```python
from build123d import *

# Parameters (mm, degrees)
TALADRO_DE_MARGEN_PARA_M101_D = 11
TALADRO_DE_MARGEN_PARA_M81_D  = 9
MATRIZC1_COUNT                = 4
CROQUIS8_R                    = 17.4
CORTAR_EXTRUIR2_DEPTH         = 70


with BuildPart() as part:
    # Croquis2 → Revolución1 (revolve)
    with BuildSketch(Plane.XY):
        with BuildLine():
            Line((19, 31), (0, 31))
            Line((0, 31), (0, 0))
            Line((0, 0), (110, 0))
            Line((110, 0), (110, 9))
            ThreePointArc((110, 9), (104.142135624, 23.142135624), (90, 29))
            Line((90, 29), (62, 29))
            Line((62, 29), (52, 23))
            Line((52, 23), (47, 3))
            Line((47, 3), (19, 3))
            Line((19, 3), (19, 31))
        make_face()
        with BuildLine():
            Line((110, 0), (0, 0))
            Line((0, 0), (0, -31))
            Line((0, -31), (19, -31))
            Line((19, -31), (19, -3))
            Line((19, -3), (47, -3))
            Line((47, -3), (52, -23))
            Line((52, -23), (62, -29))
            Line((62, -29), (90, -29))
            ThreePointArc((90, -29), (104.142135624, -23.142135624), (110, -9))
            Line((110, -9), (110, 0))
        make_face()
    revolve(axis=Axis((0, 64.768346902, 0), (0, -1, 0)))

    # Taladro de margen para M101 (through all)
    with Locations(Plane(origin=(0, 31, 0), x_dir=(1, 0, 0), z_dir=(0, 1, 0))):
        with Locations((0, 0)):
            Hole(TALADRO_DE_MARGEN_PARA_M101_D / 2)

    # Taladro de margen para M81 (through all)
    with Locations(Plane(origin=(0, 3, 0), x_dir=(1, 0, 0), z_dir=(0, 1, 0))):
        with Locations((0, 34.5)):
            taladro_de_margen_para_m81 = Hole(TALADRO_DE_MARGEN_PARA_M81_D / 2)

    # MatrizC1: Taladro de margen para M81 ×4 about axis
    matrizc1_axis = Axis((0, 0, 0), (0, 1, 0))
    for i in range(1, MATRIZC1_COUNT):
        add(taladro_de_margen_para_m81.rotate(matrizc1_axis, i * 360 / MATRIZC1_COUNT), mode=Mode.SUBTRACT)

    # Croquis8 → Cortar-Extruir2 (cut)
    with BuildSketch(Plane(origin=(0, 31, 0), x_dir=(1, 0, 0), z_dir=(0, 1, 0))):
        Circle(CROQUIS8_R)
    extrude(amount=-CORTAR_EXTRUIR2_DEPTH, mode=Mode.SUBTRACT)


solid = part.part
```
CAD build for the part. Positions are in the model's coordinates, mm. A direction names the side the tool comes from. Round coordinates to 2 decimals unless told otherwise and drop trailing zeros.
Q1. Which spindle directions (+Z, -Z, +X, -X, +Y, -Y) get a long thin tool onto all of the face, cutting with end or side? Do faces 4 (the flat face through (6, 31, -17)), 5 (the cylindrical face through (8.767, -16.804, -16.856)), 6 (the cylindrical face through (8.767, 17.196, -16.856)). Say none if no direction does.
Q2. Wall check: L1, parallel to Z at x = 0, y = -1.5; L2, parallel to Z at x = 11, y = 19; L3, parallel to Y at x = -46, z = 48. Give the ranges that are in metal, low to high.
Q3. Slice it at A-A (x = 0). State how many separate pieces and enclosed holes the cut face has, and give its area (3 significant figures).
Q4. Two-plate mould, pull along X, no slides. Class faces 1 (the cylindrical face through (-23.846, 0.126, -107.384)), 2 (the flat face through (21, -29, -59)), 3 (the conical face through (45.13, -4.25, 14.21)): pulls with the +X half, pulls with the -X half, needs draft (parallel to the pull), parting line crosses it, or undercut.
Q5. Drop flat-ended pins along their axis: pin 1 (8 mm diameter, centred on y = 13.5, z = 7, fed in from -X); pin 2 (4 mm diameter, centred on x = 66, z = 16, fed in from +Y); pin 3 (4 mm diameter, centred on y = -20, z = -30.5, fed in from +X). Give the stop position or say it passes through.
Results below:
1. face 4: +Z, -Z, +X, -X, +Y
1. face 5: -Y
1. face 6: +Y
2. L1: z = -110 to -39, -30 to -17.4, 17.4 to 30, 39 to 110
2. L2: z = -106.76 to -49.8, -15.49 to -13.48, 13.48 to 15.49, 49.8 to 106.76
2. L3: y = -29 to 29
3. separate pieces: 4
3. enclosed holes: 0
3. area: 6,950 mm2
4. face 1: parting line crosses it
4. face 2: needs draft
4. face 3: undercut
5. pin 1: stops at x = -109.86
5. pin 2: stops at y = 29
5. pin 3: stops at x = 103.61
